Part model, mm, in its own coordinate system. A direction names the side the tool comes from. Give positions to 0.01 mm unless a question says otherwise; leave off trailing zeros. Order: outer loops, then holes, each group sorted by start corner. A loop starts at its lowest first (then second) coordinate and runs counter-clockwise, first axis right, second up. Notation, with made-up numbers: (22.25, 37) - (30.25, 37) arc R28 cw to (30.25, 59) - close; hole circle Ø7 at (24.25, 32). An arc over 180 degrees is marked (long way). One line per item, written item: value.
```python
from build123d import *

# Parameters (mm, degrees)
SKETCH1_W           = 15
SKETCH1_H           = 23
SKETCH1_R           = 1.5
BOSS_EXTRUDE1_DEPTH = 2
SKETCH2_R           = 7.5
BOSS_EXTRUDE2_DEPTH = 11
SKETCH3_R           = 2.9875
BOSS_EXTRUDE3_DEPTH = 15
SKETCH4_W           = 15
SKETCH4_H           = 4.05
BOSS_EXTRUDE4_DEPTH = 2
CHAMFER1_SIZE       = 0.5
FILLET1_R           = 3


with BuildPart() as part:
    # Sketch1 → Boss-Extrude1 (new body)
    with BuildSketch(Plane.XY):
        Rectangle(SKETCH1_W, SKETCH1_H)
        with Locations((-5, 9)):
            Circle(SKETCH1_R, mode=Mode.SUBTRACT)
        with Locations(Location((5, 9, 0), (0, 0, 180))):
            Circle(SKETCH1_R, mode=Mode.SUBTRACT)
        with Locations((5, -9)):
            Circle(SKETCH1_R, mode=Mode.SUBTRACT)
        with Locations(Location((-5, -9, 0), (0, 0, 180))):
            Circle(SKETCH1_R, mode=Mode.SUBTRACT)
    extrude(amount=BOSS_EXTRUDE1_DEPTH)

    # Sketch2 → Boss-Extrude2 (add)
    with BuildSketch(Plane.XY.offset(2)):
        Circle(SKETCH2_R)
    extrude(amount=BOSS_EXTRUDE2_DEPTH)

    # Sketch3 → Boss-Extrude3 (add)
    with BuildSketch(Plane.XY.offset(13)):
        Circle(SKETCH3_R)
    extrude(amount=BOSS_EXTRUDE3_DEPTH)

    # Sketch4 → Boss-Extrude4 (add)
    with BuildSketch(Plane(origin=(0, 0, 0), x_dir=(-1, 0, 0), z_dir=(0, 0, -1))):
        Rectangle(SKETCH4_W, SKETCH4_H)
    extrude(amount=BOSS_EXTRUDE4_DEPTH)

    # Chamfer1
    chamfer1_edges = [part.edges().sort_by_distance(p)[0] for p in [
        (0, -2.025, -2),
        (0, 2.025, -2),
    ]]
    chamfer(chamfer1_edges, length=CHAMFER1_SIZE)

    # Fillet1
    fillet1_edges = [part.edges().sort_by_distance(p)[0] for p in [
        (-7.5, 11.5, 1),
        (7.5, 11.5, 1),
        (7.5, -11.5, 1),
        (-7.5, -11.5, 1),
    ]]
    fillet(fillet1_edges, radius=FILLET1_R)


solid = part.part
```
1) Cut at A-A, the plane y = -4.5. Give the cut face in (x, z), then the cut area to 3 significant figures.
Outcome:
outline: (-7.5, 0) - (7.5, 0) - (7.5, 2) - (6, 2) - (6, 13) - (-6, 13) - (-6, 2) - (-7.5, 2) - close
area: 162 mm^2
2) Cut at C-C, the plane y = -9. Give the cut face in (x, z), then the cut area to 3 significant figures.
Outcome:
outline: (-7.46, 0) - (-6.5, 0) - (-6.5, 2) - (-7.46, 2) - close; (-3.5, 0) - (3.5, 0) - (3.5, 2) - (-3.5, 2) - close; (6.5, 0) - (7.46, 0) - (7.46, 2) - (6.5, 2) - close
area: 17.8 mm^2
3) Which spindle directions (+Z, -Z, +X, -X, +Y, -Y) get a long thin tool onto all of the face, cutting with end or side? Do faces 1 (the flat face through (0, 7, 0)), 2 (the cylindrical face through (-7.493, 0.33, 7.423)), 3 (the flat face through (0, -7, 0)). Say none if no direction does.
Outcome:
face 1: -Z, +X, -X, +Y
face 2: +Z
face 3: -Z, +X, -X, -Y
4) Mould opens along Y. For faces 4 (the cylindrical face through (6.6, -10.64, 1.01)), 5 (the flat face through (0, 2.025, -1)), 6 (the cylindrical face through (-5.69, -7.67, 0.99)), 7 (the cylindrical face through (5.325, 10.464, 0.986)) say: released by +Y, released by -Y, zero draft, split by the parting line, or undercut.
Outcome:
face 4: released by -Y
face 5: released by +Y
face 6: undercut
face 7: undercut
5) Drill centre lines: line 1 along Y through (x, z) = (-5, 1.15); line 2 along Z through (x, y) = (2.75, 10); line 3 along Y through (x, z) = (6, 5.75). Where is each one in solid material? Low to high. Write a range as from..to.
Outcome:
line 1: y = -11.46..-10.5, -7.5..7.5, 10.5..11.46
line 2: z = 0..2
line 3: y = -4.5..4.5
6) Cut at B-B, the plane x = 0. Give the cut face in (y, z) (1 decimal), then the cut area to 3 significant figures.
Outcome:
outline: (-11.5, 0) - (-2, 0) - (-2, -1.5) - (-1.5, -2) - (1.5, -2) - (2, -1.5) - (2, 0) - (11.5, 0) - (11.5, 2) - (7.5, 2) - (7.5, 13) - (3, 13) - (3, 28) - (-3, 28) - (-3, 13) - (-7.5, 13) - (-7.5, 2) - (-11.5, 2) - close
area: 308 mm^2
7) Cut at D-D, the plane x = 5. Give the cut face in (y, z) (3 decimals), then the cut area to 3 significant figures.
Outcome:
outline: (-11.458, 0) - (-10.5, 0) - (-10.5, 2) - (-11.458, 2) - close; (-7.5, 0) - (-2.025, 0) - (-2.025, -1.5) - (-1.525, -2) - (1.525, -2) - (2.025, -1.5) - (2.025, 0) - (7.5, 0) - (7.5, 2) - (5.59, 2) - (5.59, 13) - (-5.59, 13) - (-5.59, 2) - (-7.5, 2) - close; (10.5, 0) - (11.458, 0) - (11.458, 2) - (10.5, 2) - close
area: 165 mm^2
8) Pin check, flat tips, straight feed: pin 1 (5 mm diameter, centred on x = -1.5, z = 18, fed in from +Y); pin 2 (3 mm diameter, centred on x = 2.5, y = 7, fed in from -Z); pin 3 (3.5 mm diameter, centred on x = -5, y = -9, fed in from +Z); pin 4 (2.5 mm diameter, centred on x = 5, y = -9, fed in from -Z). Stop position of each tip, or through.
Outcome:
pin 1: stops at y = 2.99
pin 2: stops at z = 0
pin 3: stops at z = 2
pin 4: passes through
